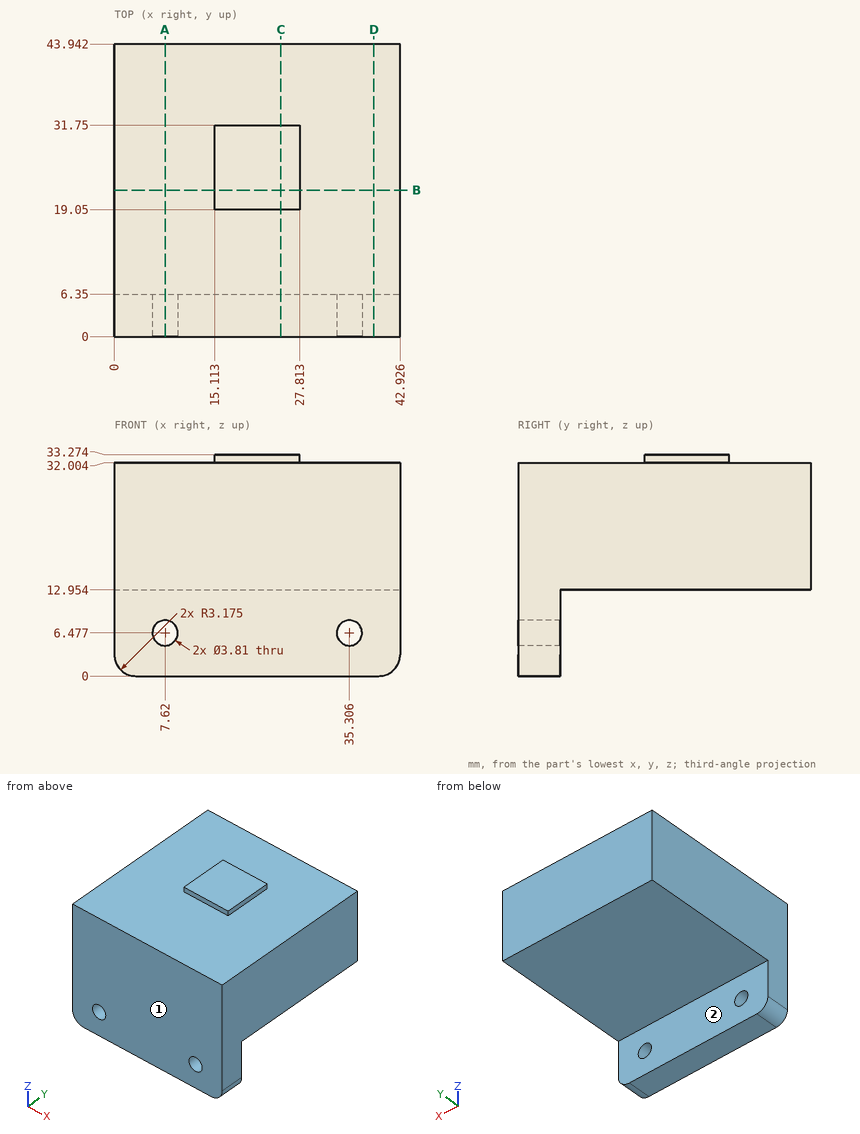
The drawing under review shows one solid part. Ordinate dimensions are in mm from its lowest x, y, z. A direction names the side the tool comes from. Give positions to 0.01 mm unless a question says otherwise; leave off trailing zeros. Write each loop counter-clockwise with the first axis right and the second up, starting at its lowest first coordinate (ties: lowest second). Pieces come first, ordered by that corner, then holes. Notation, with made-up numbers: M -14,82 L 12,82 A25 cw 12,117 Z; hole C 78,-30.75 d1. An arc over 180 degrees is marked long. Write each question's results on one line, items separated by ' | '. Start each with the question number.
1. We need section A-A (x = 7.62). Write out the cut boundary in (y, z).
2. We need section D-D (x = 39). Write out the cut boundary in (y, z), and give its area (3 significant figures).
3. We need section C-C (x = 25). Write out the cut boundary in (y, z), and give its area (3 significant figures).
4. For probe 1 along Z at (x, y) = (7.62, 2.25); probe 2 along Y at (x, z) = (26, 4); probe 3 along Z at (x, y) = (28.5, 28), list the stretches that pass through material, from the lowest coordinate up. Write a range as [from, to].
5. Insertion check: pin 1 Ø6 at (x, y) = (8.5, 39) entering from -Z; pin 2 Ø0.6 at (x, z) = (19.5, 32.5) entering from +Y; pin 3 Ø1.4 at (x, z) = (24, 33) entering from -Y. Each pin has a flat end and moves straight along its axis. Give the tip position at first contact, or say it passes through.
6. For the marked faces 1 and 2, list the 3-axis set-ups (+Z, -Z, +X, -X, +Y, -Y) from which the entire face can be reached by the end or side of a thin tool; tool diameter is ignored.
7. We need section B-B (y = 22). Write out the cut boundary in (x, z), and give its area (3 significant figures).
Results found:
1) outline: M 0,0 L 6.35,0 L 6.35,4.57 L 0,4.57 Z; M 0,8.38 L 6.35,8.38 L 6.35,12.95 L 43.94,12.95 L 43.94,32 L 0,32 Z
2) outline: M 0,0 L 6.35,0 L 6.35,12.95 L 43.94,12.95 L 43.94,32 L 0,32 Z | area: 919 mm^2
3) outline: M 0,0 L 6.35,0 L 6.35,12.95 L 43.94,12.95 L 43.94,32 L 31.75,32 L 31.75,33.27 L 19.05,33.27 L 19.05,32 L 0,32 Z | area: 935 mm^2
4) probe 1: z = [0, 4.57], [8.38, 32] | probe 2: y = [0, 6.35] | probe 3: z = [12.95, 32]
5) pin 1: stops at z = 12.95 | pin 2: stops at y = 31.75 | pin 3: stops at y = 19.05
6) face 1: +Z, -Z, +X, -X, -Y | face 2: -Z, +X, -X, +Y
7) outline: M 0,12.95 L 42.93,12.95 L 42.93,32 L 27.81,32 L 27.81,33.27 L 15.11,33.27 L 15.11,32 L 0,32 Z | area: 834 mm^2
